Part model, mm, in its own coordinate system. Face numbers are marked on the shaded views. A direction names the side the tool comes from. Coordinates: 2 decimals unless noted, no trailing zeros. Order: outer loops, then holes, each group sorted by start corner. A loop starts at its lowest first (then second) coordinate and runs counter-clockwise, first axis right, second up.
from build123d import *

# Parameters (mm, degrees)
PAD_DEPTH            = 20
SKETCH001_R          = 25
POCKET_DEPTH         = 18.001
POCKET_DEPTH_BACK    = -18.001
POCKET001_DEPTH      = 9.5
POCKET002_DEPTH      = 3
POCKET002_DEPTH_BACK = -55
POCKET003_DEPTH      = 4.5
SKETCH006_W          = 30.00024
SKETCH006_H          = 49.987866
POCKET004_DEPTH      = 20.001
POCKET004_DEPTH_BACK = -20.001


with BuildPart() as part:
    # Sketch → Pad (new body, symmetric)
    with BuildSketch(Plane.XZ):
        with BuildLine():
            ThreePointArc((0, 18), (-18, 0), (0, -18))
            Line((0, -18), (50, -18))
            ThreePointArc((50, -18), (68, 0), (50, 18))
            Line((0, 18), (50, 18))
        make_face()
    extrude(amount=PAD_DEPTH, both=True)

    # Sketch001 → Pocket (cut, two sides)
    with BuildSketch(Plane.XY) as pocket_sk:
        with Locations((-35, 0)):
            Circle(SKETCH001_R)
        with Locations((85, 0)):
            Circle(SKETCH001_R)
    extrude(amount=-POCKET_DEPTH, mode=Mode.SUBTRACT)
    extrude(pocket_sk.sketch, amount=-POCKET_DEPTH_BACK, mode=Mode.SUBTRACT)

    # Sketch002 (on DatumPlane) → Pocket001 (cut, symmetric)
    with BuildSketch(Plane.XY):
        with BuildLine():
            ThreePointArc((-11.5, -14.282857), (-7.5, 0), (-11.5, 14.282857))
            Line((-11.5, 20), (-11.5, 14.282857))
            Line((-11.5, 20), (55, 20))
            Line((55, 20), (55, -20))
            Line((-11.5, -20), (55, -20))
            Line((-11.5, -14.282857), (-11.5, -20))
        make_face()
    extrude(amount=POCKET001_DEPTH, both=True, mode=Mode.SUBTRACT)

    # Sketch003 (on DatumPlane) → Pocket002 (cut, two sides)
    with BuildSketch(Plane.YZ) as pocket002_sk:
        Polygon((-20, 9), (-16, 15), (16, 15), (20, 9), (20, -9), (16, -15), (-16, -15), (-20, -9), align=None)
    extrude(amount=-POCKET002_DEPTH, mode=Mode.SUBTRACT)
    extrude(pocket002_sk.sketch, amount=-POCKET002_DEPTH_BACK, mode=Mode.SUBTRACT)

    # Sketch005 (on DatumPlane) → Pocket003 (cut)
    with BuildSketch(Plane.YZ.offset(-2)):
        Polygon((-17, 16), (-2, 16), (1, 9.5), (-20, 9.5), align=None)
        Polygon((-1, -9.5), (20, -9.5), (17, -16), (2, -16), align=None)
    extrude(amount=-POCKET003_DEPTH, mode=Mode.SUBTRACT)

    # Sketch006 → Pocket004 (cut, two sides)
    with BuildSketch(Plane.XZ) as pocket004_sk:
        with Locations((68.822588, 0.861696)):
            Rectangle(SKETCH006_W, SKETCH006_H)
    extrude(amount=-POCKET004_DEPTH, mode=Mode.SUBTRACT)
    extrude(pocket004_sk.sketch, amount=-POCKET004_DEPTH_BACK, mode=Mode.SUBTRACT)


solid = part.part
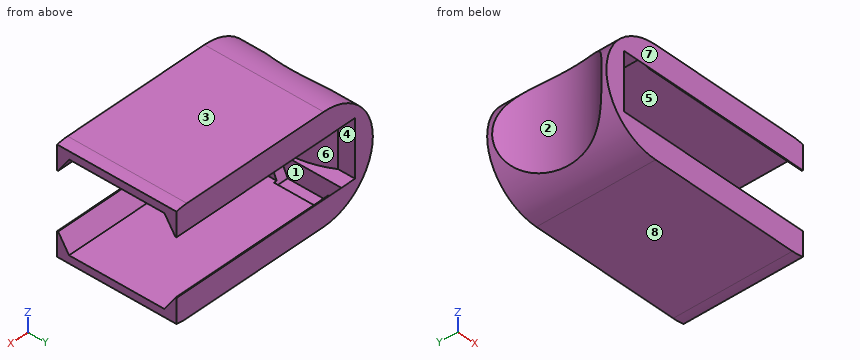
Q1. Cut at C-C on y = 3.5. Write the cut outline in (x, z), and give its area (3 significant figures).
Results list:
outline: (-10.25, -14.8) arc R18 ccw to (0, -18) - (50, -18) arc R18 ccw to (53.82, -17.59) - (53.82, -15) - (-2, -15) - (-2, -16) - (-6.5, -16) - (-6.5, -9.5) - (-7.72, -9.5) - (-7.72, 9.5) - (-3, 9.5) - (-3, 15) - (53.82, 15) - (53.82, 17.59) arc R18 ccw to (50, 18) - (0, 18) arc R18 ccw to (-10.25, 14.8) - close
area: 466 mm2
Q2. Pin check, flat tips, straight feed: pin 1 Ø8 at (x, z) = (4.5, -6.5) entering from -Y; pin 2 Ø5 at (y, z) = (7, -13.5) entering from -X; pin 3 Ø1.3 at (x, y) = (-5.5, -9) entering from -Z; pin 4 Ø6 at (y, z) = (8, 11) entering from +X. Stop position of each tip, or through.
Results list:
pin 1: stops at y = -20
pin 2: stops at x = -11.88
pin 3: stops at z = -17.33
pin 4: stops at x = -3
Q3. Cut at B-B on z = 0. Write the cut outline in (x, y), and give its area (3 significant figures).
Results list:
outline: (-18, -20) - (-11.5, -20) - (-11.5, -14.28) arc R27.5 ccw to (-11.5, 14.28) - (-11.5, 20) - (-18, 20) - (-18, 18.33) arc R25 cw to (-18, -18.33) - close
area: 135 mm2
Q4. Mould opens along Z. For the marked faces 6, 7 and 8 say: pulls with the +Z half, pulls with the -Z half, needs draft (parallel to the pull), parting line crosses it, or undercut.
Results list:
face 6: undercut
face 7: needs draft
face 8: pulls with the -Z half
Q5. Cut at A-A on x = 23.5. Write the cut outline in (y, z), and give its area (3 significant figures).
Results list:
outline: (-20, -18) - (20, -18) - (20, -9.5) - (19.67, -9.5) - (16, -15) - (-16, -15) - (-19.67, -9.5) - (-20, -9.5) - close; (-20, 9.5) - (-19.67, 9.5) - (-16, 15) - (16, 15) - (19.67, 9.5) - (20, 9.5) - (20, 18) - (-20, 18) - close
area: 288 mm2
Q6. Which spindle directions (+Z, -Z, +X, -X, +Y, -Y) get a long thin tool onto all of the face, cutting with end or side? Do the marked faces 1, 2, 3, 4 and 5. Say none if no direction does.
Results list:
face 1: none
face 2: +Z, -Z, -X
face 3: +Z, +X, -X, +Y, -Y
face 4: +X, +Y
face 5: +X
Q7. Wall check: line 1 along Z through (x, y) = (11, -11.5); line 2 along Y through (x, z) = (1, 11.5); line 3 along Y through (x, z) = (19.5, 12). Give the ranges that are in metal, low to high.
Results list:
line 1: z = -18 to -15, 15 to 18
line 2: y = -20 to -18.33, 18.33 to 20
line 3: y = -20 to -18, 18 to 20
Q8. Cut at D-D on z = 8. Write the cut outline in (x, y), and give its area (3 significant figures).
Results list:
outline: (-16.12, -20) - (-11.5, -20) - (-11.5, -14.28) arc R27.5 ccw to (-11.5, 14.28) - (-11.5, 20) - (-16.12, 20) - (-16.12, 16.39) arc R25 cw to (-16.12, -16.39) - close
area: 125 mm2
